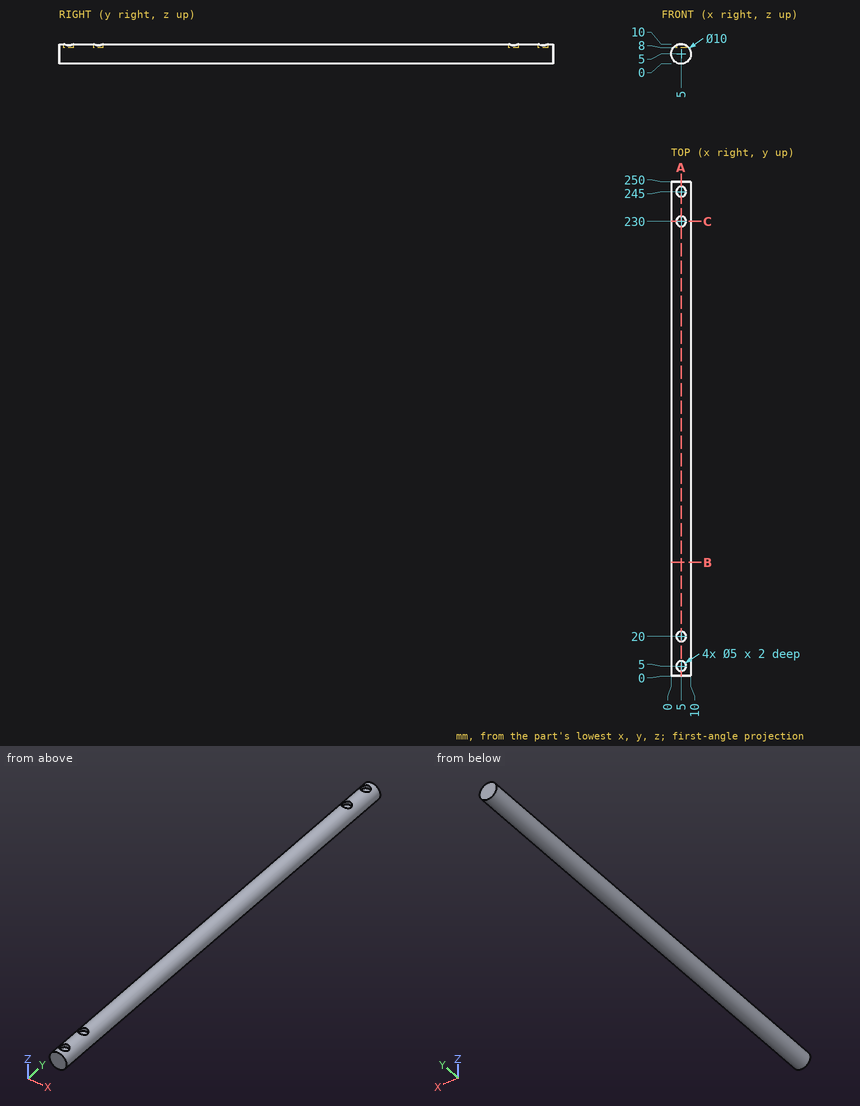
Check sheet for the drawn part. Datum: minimum x, y, z corner. Units: mm. Round coordinates to 2 decimals unless told otherwise and drop trailing zeros. Loops run counter-clockwise (first coordinate to the right, second up) from the corner with the lowest first, then second, coordinate; pieces in that order, holes last. Notation, with made-up numbers: (77.5, -24) - (124.5, -24) arc R32 cw to (124.5, 12) - close; hole circle Ø2 at (43, 43.5). An arc over 180 degrees is marked (long way). Answer as a JSON object with one key per item and string values. Group by question number.
Q1. Sectioned sample at C-C, the plane y = 230. Enter the section's corners in (x, z), plus the area to 3 significant figures.
Q2. Sectioned sample at B-B, the plane y = 57.5. Enter the section's corners in (x, z).
Q3. Sectioned sample at A-A, the plane x = 5. Enter the section's corners in (y, z), plus the area to 3 significant figures.
Q4. Gauge pin test, flat ends, axial feed: P1, Ø2.5, axis at x = 4.5, y = 229, coming from the +Z side; P2, Ø4, axis at x = 2, y = 191.5, coming from the -Z side. Record the tip position at first contact, or that the pin passes through.
Q5. Scan lines: line 1 along Y through (x, z) = (5, 9.35); line 2 along Z through (x, y) = (5.5, 139). Record each from-to range of solid material in increasing order. Write a range as [from, to].
Solution:
{
 "1": {"outline": "(2.5, 8) - (2.5, 9.33) arc R5 ccw (long way) to (7.5, 9.33) - (7.5, 8) - close", "area": "69.6 mm²"},
 "2": {"outline": "circle Ø10 at (5, 5)"},
 "3": {"outline": "(0, 0) - (250, 0) - (250, 10) - (247.5, 10) - (247.5, 8) - (242.5, 8) - (242.5, 10) - (232.5, 10) - (232.5, 8) - (227.5, 8) - (227.5, 10) - (22.5, 10) - (22.5, 8) - (17.5, 8) - (17.5, 10) - (7.5, 10) - (7.5, 8) - (2.5, 8) - (2.5, 10) - (0, 10) - close", "area": "2,460 mm²"},
 "4": {"P1": "stops at z = 8", "P2": "stops at z = 0.1"},
 "5": {"line 1": "y = [0, 2.5], [7.5, 17.5], [22.5, 227.5], [232.5, 242.5], [247.5, 250]", "line 2": "z = [0.03, 9.97]"}
}
